Here's how the part is built. I have some questions about the finished solid (model axes, mm). Coordinates: 2 decimals unless noted, no trailing zeros. Loops run counter-clockwise (first coordinate to the right, second up) from the corner with the lowest first, then second, coordinate; pieces in that order, holes last.
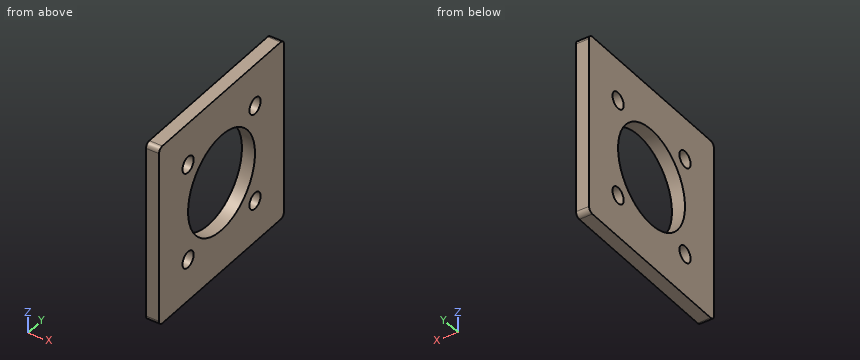
```python
from build123d import *

# Parameters (mm, degrees)
F0_W     = 56
F0_H     = 56
F0_R     = 2.5
F0_R_2   = 15
F1_DEPTH = 4
F2_R     = 1.5


# Not quite as in the source:
# - a feature names something its author has since deleted; it is built from what else it names


with BuildPart() as f1:
    # F0 (on Right) → F1 (new body)
    with BuildSketch(Plane.YZ):
        Rectangle(F0_W, F0_H)
        with Locations((-15, -15)):
            Circle(F0_R, mode=Mode.SUBTRACT)
        with Locations((15, -15)):
            Circle(F0_R, mode=Mode.SUBTRACT)
        with Locations((-15, 15)):
            Circle(F0_R, mode=Mode.SUBTRACT)
        Circle(F0_R_2, mode=Mode.SUBTRACT)
        with Locations((15, 15)):
            Circle(F0_R, mode=Mode.SUBTRACT)
    extrude(amount=F1_DEPTH)

    # F2
    f2_edges = [f1.edges().sort_by_distance(p)[0] for p in [
        (2, -28, 28),
        (2, -28, -28),
        (2, 28, -28),
        (2, 28, 28),
    ]]
    fillet(f2_edges, radius=F2_R)


with BuildPart() as f3_1:
    # F3: copy of F1
    add(f1.part)


solid = f1.part
```
1. For pin 1 (1.5 mm diameter, centred on y = 15, z = -15, fed in from -X), with a flat end and sliding along its axis, tell me the tip position at first contact or that it passes through.
2. I want a section at D-D (y = -13.5). Please give me the cut outline in (x, z).
3. I want a section at A-A (z = -1.5). Please give me the cut outline in (x, y).
4. I want a section at B-B (y = 0). Please give me the cut outline in (x, z).
5. I need wall thicknesses on line 1 along Z through (x, y) = (2.4, -13.5); line 2 along Y through (x, z) = (3.6, 4.5); line 3 along Y through (x, z) = (3.5, -1). Which ranges of each line are inside material? Lowest first, please.
6. I want a section at C-C (x = 1.35). Please give me the cut outline in (y, z).
Response values:
1. pin 1: passes through
2. outline: (0, -28) - (4, -28) - (4, -17) - (0, -17) - close; (0, -13) - (4, -13) - (4, -6.54) - (0, -6.54) - close; (0, 6.54) - (4, 6.54) - (4, 13) - (0, 13) - close; (0, 17) - (4, 17) - (4, 28) - (0, 28) - close
3. outline: (0, -28) - (4, -28) - (4, -14.92) - (0, -14.92) - close; (0, 14.92) - (4, 14.92) - (4, 28) - (0, 28) - close
4. outline: (0, -28) - (4, -28) - (4, -15) - (0, -15) - close; (0, 15) - (4, 15) - (4, 28) - (0, 28) - close
5. line 1: z = -28 to -17, -13 to -6.54, 6.54 to 13, 17 to 28
5. line 2: y = -28 to -14.31, 14.31 to 28
5. line 3: y = -28 to -14.97, 14.97 to 28
6. outline: (-28, -26.5) arc R1.5 ccw to (-26.5, -28) - (26.5, -28) arc R1.5 ccw to (28, -26.5) - (28, 26.5) arc R1.5 ccw to (26.5, 28) - (-26.5, 28) arc R1.5 ccw to (-28, 26.5) - close; hole circle Ø5 at (-15, -15); hole circle Ø5 at (-15, 15); hole circle Ø30 at (0, 0); hole circle Ø5 at (15, -15); hole circle Ø5 at (15, 15)
